```python
from build123d import *

# Parameters (mm, degrees)
BASE_FLANGE3_DEPTH = 50
SKETCH21_R         = 1.65
CUT_EXTRUDE1_DEPTH = 3
CIRPATTERN1_COUNT  = 4
SKETCH22_R         = 2.15
CUT_EXTRUDE4_DEPTH = 60
CUT_EXTRUDE3_START = -60
SKETCH23_R         = 2.15
CUT_EXTRUDE3_DEPTH = 60


# Read off the part's stored shape, not the designer's step: Base-Flange3
with BuildPart() as part:
    # Base-Flange3 outline → Base-Flange3 (new body)
    with BuildSketch(Plane.XY):
        with BuildLine():
            Line((-30.25, 24.5), (-30.25, -29))
            Line((-30.25, -29), (-25.25, -29))
            Line((-25.25, -29), (-25.25, 24.5))
            ThreePointArc((-25.25, 24.5), (-25.103553391, 24.853553391), (-24.75, 25))
            Line((-24.75, 25), (24.75, 25))
            ThreePointArc((24.75, 25), (25.103553391, 24.853553391), (25.25, 24.5))
            Line((25.25, 24.5), (25.25, -29))
            Line((25.25, -29), (30.25, -29))
            Line((30.25, -29), (30.25, 24.5))
            ThreePointArc((30.25, 24.5), (28.639087297, 28.389087297), (24.75, 30))
            Line((24.75, 30), (-24.75, 30))
            ThreePointArc((-24.75, 30), (-28.639087297, 28.389087297), (-30.25, 24.5))
        make_face()
    extrude(amount=BASE_FLANGE3_DEPTH)

    # Sketch21 → Cut-Extrude1 (cut)
    with BuildSketch(Plane.XZ.offset(-25)):
        with Locations(Location((-15, 40, 0), (0, 0, 270))):
            Circle(SKETCH21_R)
    cut_extrude1 = extrude(amount=-CUT_EXTRUDE1_DEPTH, mode=Mode.SUBTRACT)

    # CirPattern1: Cut-Extrude1 ×4 about axis
    cirpattern1_axis = Axis((0.052016033, 0, 24.947983967), (0, 1, 0))
    for i in range(1, CIRPATTERN1_COUNT):
        add(cut_extrude1.rotate(cirpattern1_axis, i * 360 / CIRPATTERN1_COUNT), mode=Mode.SUBTRACT)

    # Sketch22 → Cut-Extrude4 (cut)
    with BuildSketch(Plane.ZY.offset(30.25)):
        with Locations(Location((12.5, -4, 0), (0, 0, 270))):
            Circle(SKETCH22_R)
    cut_extrude4 = extrude(amount=-CUT_EXTRUDE4_DEPTH, mode=Mode.SUBTRACT)

    # Mirror2: Cut-Extrude4 across plane
    add(cut_extrude4.mirror(Plane.XY.offset(25)), mode=Mode.SUBTRACT)

    # Sketch23 → Cut-Extrude3 (cut)
    with BuildSketch(Plane(origin=(30.25, 0, 0), x_dir=(0, 0, -1), z_dir=(1, 0, 0)).offset(CUT_EXTRUDE3_START)):
        with Locations(Location((-25.574194975, -4, 0), (0, 0, 90))):
            Circle(SKETCH23_R)
        with Locations(Location((-37.5, -4, 0), (0, 0, 270))):
            Circle(SKETCH23_R)
    extrude(amount=CUT_EXTRUDE3_DEPTH, mode=Mode.SUBTRACT)


solid = part.part
```
CAD build for the part. Positions are in the model's coordinates, mm. A direction names the side the tool comes from. Coordinates: 2 decimals unless noted, no trailing zeros. Order: outer loops, then holes, each group sorted by start corner. A loop starts at its lowest first (then second) coordinate and runs counter-clockwise, first axis right, second up. Notation, with made-up numbers: M -29,-21 L -8,-21 A8 cw -8,-14 Z; hole C 85,-10.5 d9. An arc over 180 degrees is marked long. Answer as CSV lines item,"result".
1) Cut at B-B (y = -7.5). List the corners of the cut face in (x, z), then the cut area to 3 significant figures.
Verdict:
outline,"M -30.25,0 L -25.25,0 L -25.25,50 L -30.25,50 Z; M 25.25,0 L 30.25,0 L 30.25,50 L 25.25,50 Z"
area,"500 mm2"
2) Cut at D-D (x = 26.5). List the corners of the cut face in (y, z).
Verdict:
outline,"M -29,0 L 29.71,0 L 29.71,50 L -29,50 Z; hole C -4,12.5 d4.3; hole C -4,25.57 d4.3; hole C -4,37.5 d4.3"
3) Mould opens along Z. For faces 4 (the cylindrical face through (-27.53, -5.58, 27.03)), 5 (the flat face through (-5, 27, 0)), 6 (the flat face through (0, 30, 25)) say: released by +Z, released by -Z, zero draft, split by the parting line, or undercut.
Verdict:
face 4,"undercut"
face 5,"released by -Z"
face 6,"zero draft"
4) 3-axis set-ups, long thin cutter, end or side, ignore diameter. For faces 1 (the flat face through (15, 28, 10)), 2 (the flat face through (0, 25, 25)), 3 (the flat face through (29.75, -4, 13)): which of +Z, -Z, +X, -X, +Y, -Y reach the whole face in a straight line?
Verdict:
face 1,"-Y"
face 2,"+Z, -Z, -Y"
face 3,"-X"
5) Drill centre lines: L1, parallel to Z at x = -26.65, y = -4; L2, parallel to X at y = 21, z = 25.5; L3, parallel to Y at x = -10, z = 34.5. Where is each one in solid material? Low to high. Write a range as from..to.
Verdict:
L1,"0..10.35, 14.65..23.42, 27.72..35.35, 39.65..50"
L2,"-30.25..-25.25, 25.25..30.25"
L3,"25..30"
6) Flat gauge pins, fed straight in: P1, Ø25, axis at x = -3, z = 37, coming from the -Y side; P2, Ø3, axis at x = 15.1, z = 40, coming from the -Y side. Where does each tip first touch, or does it go through?
Verdict:
P1,"y = 25"
P2,"y = 28"
7) Cut at C-C (z = 37.5). List the corners of the cut face in (x, y).
Verdict:
outline,"M -30.25,-29 L -25.25,-29 L -25.25,-6.15 L -30.25,-6.15 Z; M -30.25,-1.85 L -25.25,-1.85 L -25.25,24.5 A0.5 cw -24.75,25 L 24.75,25 A0.5 cw 25.25,24.5 L 25.25,-1.85 L 30.25,-1.85 L 30.25,24.5 A5.5 ccw 24.75,30 L -24.75,30 A5.5 ccw -30.25,24.5 Z; M 25.25,-29 L 30.25,-29 L 30.25,-6.15 L 25.25,-6.15 Z"
8) Cut at A-A (z = 12.5). List the corners of the cut face in (x, y).
Verdict:
outline,"M -30.25,-29 L -25.25,-29 L -25.25,-6.15 L -30.25,-6.15 Z; M -30.25,-1.85 L -25.25,-1.85 L -25.25,24.5 A0.5 cw -24.75,25 L 24.75,25 A0.5 cw 25.25,24.5 L 25.25,-1.85 L 29.75,-1.85 L 29.75,-6.15 L 25.25,-6.15 L 25.25,-29 L 30.25,-29 L 30.25,24.5 A5.5 ccw 24.75,30 L -24.75,30 A5.5 ccw -30.25,24.5 Z"
